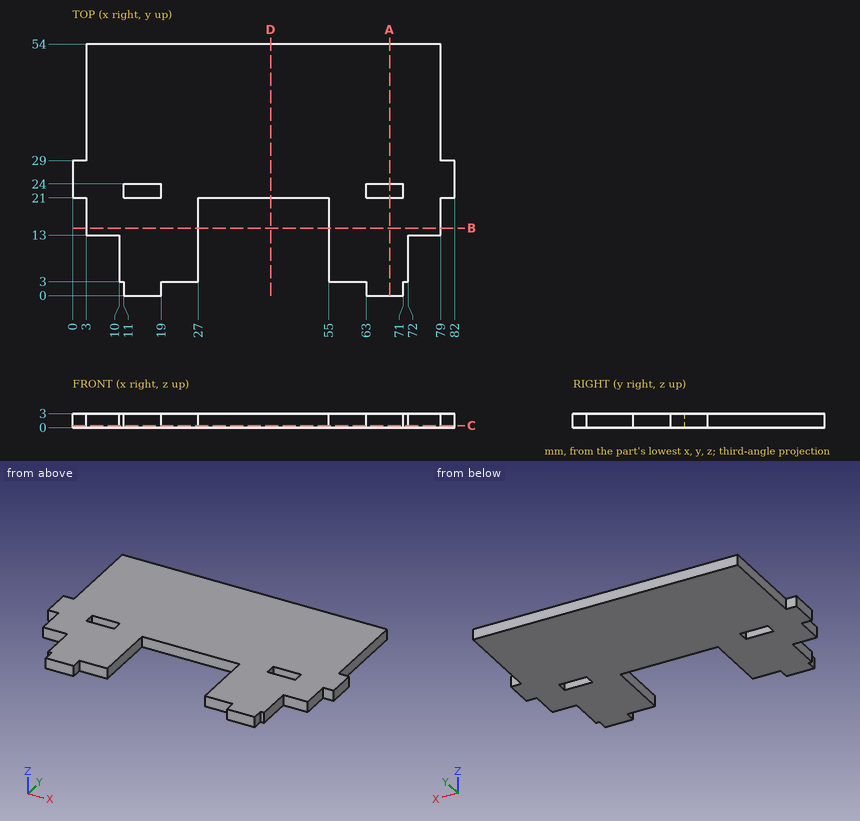
Could you check a few things on this drawing? It's one solid part, dimensions in mm from its lowest x, y, z. Coordinates: 2 decimals unless noted, no trailing zeros. Order: outer loops, then holes, each group sorted by start corner. A loop starts at its lowest first (then second) coordinate and runs counter-clockwise, first axis right, second up. Notation, with made-up numbers: (25, 59) - (78, 59) arc R18 cw to (78, 66) - close; hole circle Ø4 at (-33, 56.25). An arc over 180 degrees is marked (long way). One line per question, with ' | ' between items. Start each with the question number.
1. If we section it at A-A (x = 68): Write out the boundary of the cut face in (y, z).
2. I'm going to push flat-ended pins straight in: pin 1 Ø0.9 at (x, z) = (1, 1) entering from +Y; pin 2 Ø1.5 at (y, z) = (1.5, 2) entering from +X; pin 3 Ø0.9 at (y, z) = (41, 2) entering from +X; pin 4 Ø8 at (x, y) = (48, 14) entering from -Z. Where does each tip first touch, or does it pass through?
3. If we section it at C-C (z = 0.45): Give the number of separate pieces and of enclosed holes in the cut face, and give its area (3 significant figures).
4. If we section it at D-D (x = 42.5): Write out the boundary of the cut face in (y, z), and give its area (3 significant figures).
5. Please list where these lines run through material, in increasing order: line 1 along X through (y, z) = (17, 0.3); line 2 along Y through (x, z) = (12, 1.85); line 3 along X through (y, z) = (8, 0.5). Write a range as [from, to].
6. If we section it at B-B (y = 14.5): Write out the boundary of the cut face in (x, z).
Model answer:
1) outline: (0, 0) - (21, 0) - (21, 3) - (0, 3) - close; (24, 0) - (54, 0) - (54, 3) - (24, 3) - close
2) pin 1: stops at y = 29 | pin 2: stops at x = 71 | pin 3: stops at x = 79 | pin 4: passes through
3) separate pieces: 1 | enclosed holes: 2 | area: 3,280 mm²
4) outline: (21, 0) - (54, 0) - (54, 3) - (21, 3) - close | area: 99.0 mm²
5) line 1: x = [3, 27], [55, 79] | line 2: y = [0, 21], [24, 54] | line 3: x = [10, 27], [55, 72]
6) outline: (3, 0) - (27, 0) - (27, 3) - (3, 3) - close; (55, 0) - (79, 0) - (79, 3) - (55, 3) - close
